Can you work these out from the drawing? Everything is in mm from the part's minimum corner. A direction names the side the tool comes from. Round coordinates to 2 decimals unless told otherwise and drop trailing zeros. Order: outer loops, then holes, each group sorted by start corner. A loop starts at its lowest first (then second) coordinate and runs counter-clockwise, first axis right, second up. Notation, with made-up numbers: (67.5, 41.5) - (94.5, 41.5) arc R22 ccw to (94.5, 67.5) - close; hole circle Ø6 at (60.5, 84). An arc over 180 degrees is marked (long way). Write item = value, one per line.
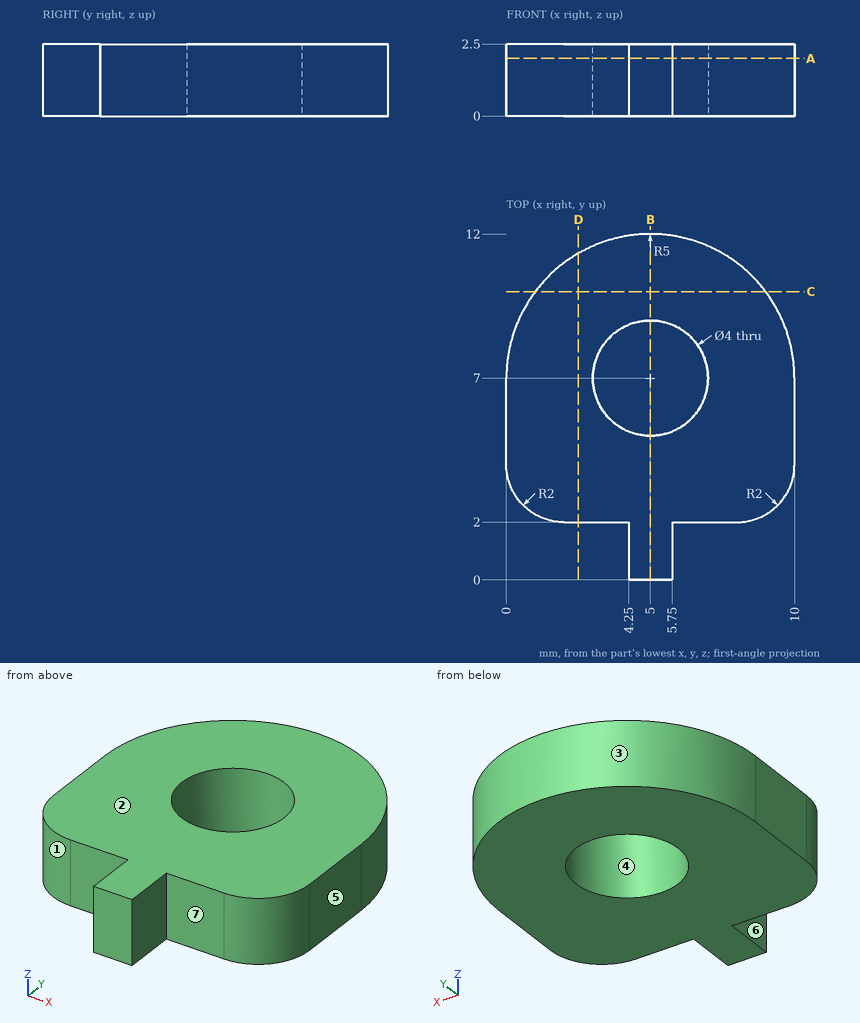
(1) If we section it at C-C (y = 10): Write out the boundary of the cut face in (x, z).
Computed:
outline = (1, 0) - (9, 0) - (9, 2.5) - (1, 2.5) - close
(2) Thinking about a two-plate mould opening in Y: for the marked faces 1, 2, 3 and 4, which applies, +Y half, -Y half, draft (parallel to the pull), parting line (faces both ways), or undercut?
Computed:
face_1 = -Y half
face_2 = draft
face_3 = +Y half
face_4 = undercut
(3) If we section it at B-B (x = 5): Write out the boundary of the cut face in (y, z), plus the area to 3 significant figures.
Computed:
outline = (0, 0) - (5, 0) - (5, 2.5) - (0, 2.5) - close; (9, 0) - (12, 0) - (12, 2.5) - (9, 2.5) - close
area = 20.0 mm^2
(4) If I drill on line 1 (X direction, y = 7, z = 2.05); line 2 (Y direction, x = 5, z = 1.55); line 3 (X direction, y = 7.75, z = 1.6), over which ranges is the centre line in solid material (lowest first)? Write a range as from..to.
Computed:
line_1 = 0..3, 7..10
line_2 = 0..5, 9..12
line_3 = 0.06..3.15, 6.85..9.94
(5) If we section it at A-A (z = 2): Write out the boundary of the cut face in (x, y).
Computed:
outline = (0, 4) arc R2 ccw to (2, 2) - (4.25, 2) - (4.25, 0) - (5.75, 0) - (5.75, 2) - (8, 2) arc R2 ccw to (10, 4) - (10, 7) arc R5 ccw to (0, 7) - close; hole circle Ø4 at (5, 7)
(6) Will these pins go through, and if not, where does the flat tip stop? P1, Ø1, axis at y = 8, z = 2, coming from the -X side; P2, Ø0.6, axis at y = 1, z = 1, coming from the +X side; P3, Ø1, axis at x = 1, z = 1, coming from the +Y side.
Computed:
P1 = 0.03
P2 = 5.75
P3 = 10.57
(7) If we section it at D-D (x = 2.5): Write out the boundary of the cut face in (y, z).
Computed:
outline = (2, 0) - (11.33, 0) - (11.33, 2.5) - (2, 2.5) - close
(8) On a 3-axis mill with a long thin cutter (end or side, diameter ignored), from which of +Z, -Z, +X, -X, +Y, -Y can I reach the whole of each face in a straight line? I mean the marked faces 5, 6 and 7. Say none if no direction works.
Computed:
face_5 = +Z, -Z, +X, +Y, -Y
face_6 = +Z, -Z, -X, -Y
face_7 = +Z, -Z, +X, -Y
